Geometry check sheet. Reference: the model listing, model coordinates, mm. Coordinates: 2 decimals unless noted, no trailing zeros. Write each loop counter-clockwise with the first axis right and the second up, starting at its lowest first coordinate (ties: lowest second). Pieces come first, ordered by that corner, then holes. Notation, with made-up numbers: M -34,-9.75 L -29,-9.75 A25 ccw -29,21.25 Z; hole C 43,-14 d10. An arc over 180 degrees is marked long. Write each question's results on one line, items separated by ' | '.
```python
from build123d import *

# Parameters (mm, degrees)
THREADSCHEMATIC_START     = -8.2042
THREADSCHEMATIC_OUTLINE_R = 5.35813
THREADSCHEMATIC_DEPTH     = 8.2042


# Read off the part's stored shape, not the designer's step: ThreadSchematic
with BuildPart() as part:
    # ThreadSchematic outline → ThreadSchematic (new body)
    with BuildSketch(Plane.XY.offset(THREADSCHEMATIC_START)):
        Polygon((9.525, 5.499261314), (0, 10.998522628), (-9.525, 5.499261314), (-9.525, -5.499261314), (0, -10.998522628), (9.525, -5.499261314), align=None)
        Circle(THREADSCHEMATIC_OUTLINE_R, mode=Mode.SUBTRACT)
    extrude(amount=THREADSCHEMATIC_DEPTH)

    # Sketch3 → Double-Chamfer (revolve, cut)
    with BuildSketch(Plane(origin=(0, 0, 0), x_dir=(0, 0, -1), z_dir=(1, 0, 0))):
        Polygon((8.2042, 9.525), (6.9342, 10.998522628), (6.9342, 23.698522628), (20.9042, 23.698522628), (20.9042, 9.525), align=None)
        Polygon((1.27, 23.698522628), (-12.7, 23.698522628), (-12.7, 9.525), (0, 9.525), (1.27, 10.998522628), align=None)
    revolve(axis=Axis((0, 0, 0), (0, 0, -1)), mode=Mode.SUBTRACT)

    # EndChamferSke → EndChamfer (revolve, cut)
    with BuildSketch(Plane(origin=(0, 0, 0), x_dir=(0, 0, -1), z_dir=(1, 0, 0)), mode=Mode.PRIVATE) as endchamfer_sk:
        Polygon((8.1788, 6.35), (7.414833664, 5.258943), (8.2296, 5.258943), (8.2296, 6.35), align=None)
        Polygon((-0.0508, 6.35), (0, 6.35), (0.763966336, 5.258943), (-0.0508, 5.258943), align=None)
    revolve(endchamfer_sk.sketch.rotate(Axis((0, 0, -25.037505729), (0, 0, -1)), 90), axis=Axis((0, 0, -25.037505729), (0, 0, -1)), mode=Mode.SUBTRACT)


solid = part.part
```
Q1. Scan lines: probe 1 along Y at (x, z) = (0.25, -5); probe 2 along X at (y, z) = (-3.25, -3) (3 decimals); probe 3 along X at (y, z) = (1.25, -6.25) (3 decimals). Record each from-to range of solid material in increasing order.
Geometry check:
probe 1: y = -10.85 to -5.35, 5.35 to 10.85 | probe 2: x = -9.525 to -4.26, 4.26 to 9.525 | probe 3: x = -9.525 to -5.21, 5.21 to 9.525
Q2. Mould release check, pull along Y, two halves, no side actions. Record for faces 1 (the flat face through (9.525, 0, -4)), 2 (the cylindrical face through (2.472, -4.754, -4.137)), 3 (the conical face through (0.024, -9.883, -0.309)), 4 (the flat face through (-4.696, 8.287, -4.16)): pulls with the +Y half, pulls with the -Y half, needs draft (parallel to the pull), parting line crosses it, or undercut.
Geometry check:
face 1: needs draft | face 2: undercut | face 3: pulls with the -Y half | face 4: pulls with the +Y half
Q3. Sectioned sample at A-A on z = -3.5. Record the cut outline in (x, y) (3 decimals), and give its area (3 significant figures).
Geometry check:
outline: M -9.525,-5.499 L 0,-10.999 L 9.525,-5.499 L 9.525,5.499 L 0,10.999 L -9.525,5.499 Z; hole C 0,0 d10.716 | area: 224 mm2
Q4. Sectioned sample at B-B on z = -1. Record the cut outline in (x, y) (1 decimal).
Geometry check:
outline: M -9.5,-4.8 A10.7 ccw -9,-5.8 L -0.6,-10.7 A10.7 ccw 0.6,-10.7 L 9,-5.8 A10.7 ccw 9.5,-4.8 L 9.5,4.8 A10.7 ccw 9,5.8 L 0.6,10.7 A10.7 ccw -0.6,10.7 L -9,5.8 A10.7 ccw -9.5,4.8 Z; hole C 0,0 d10.7
Q5. Depth check by flat-ended pin: P1, Ø1.5, axis at x = 5, z = -2, coming from the +Y side; P2, Ø1, axis at y = 8, z = -6, coming from the +X side; P3, Ø2, axis at x = 4, z = -1.5, coming from the +Y side. Enter the tip coordinate at first touch or a pass-through.
Geometry check:
P1: stops at y = 8.54 | P2: stops at x = 6.06 | P3: stops at y = 9.27
